Verification items for the finished model (mm, model axes). A direction names the side the tool comes from. Coordinates: 2 decimals unless noted, no trailing zeros. Loops run counter-clockwise (first coordinate to the right, second up) from the corner with the lowest first, then second, coordinate; pieces in that order, holes last. Notation, with made-up numbers: (12, 87.25) -> (46, 87.25) arc R23 ccw to (46, 95.25) -> close; hole circle Ø4 at (52.25, 61.25). An arc over 180 degrees is marked (long way). Write item = value, one per line.
```python
from build123d import *

# Parameters (mm, degrees)
F0_R         = 9.375
F1_DEPTH     = 140
F2_DEPTH     = 50
F3_SIZE      = 24
F4_T4_DEPTH  = 38.941125497
F4_T10_DEPTH = 38.941125497
F5_COUNT     = 3
F0_R_2       = 2.25
F6_DEPTH     = 10
F7_START     = 69.5
F0_R_3       = 7.5
F7_DEPTH     = 2.5
F8_DEPTH     = 25
F9_R         = 2
F10_DEPTH    = 25


# Not quite as in the source:
# - a fillet or chamfer that OpenCascade refuses, or shapes differently, is made with other operations: its cross-section is extruded or revolved along the edge and cut away or added


with BuildPart() as f1:
    # F0 (on Top) → F1 (new body)
    with BuildSketch(Plane.XY):
        with BuildLine():
            ThreePointArc((3, -9.801147892), (8.2405248619, -6.0955926701), (10.25, 0))
            ThreePointArc((10.25, 0), (7.5083287088, 6.9776428685), (0.75, 10.2225241501))
            ThreePointArc((0.75, 10.2225241501), (0, 10.25), (-0.75, 10.2225241501))
            ThreePointArc((-0.75, 10.2225241501), (-10.185896402, 1.1445586432), (-3, -9.801147892))
            ThreePointArc((-3, -9.801147892), (-1.5166961062, -10.1371659216), (-1.65e-08, -10.25))
            ThreePointArc((-1.65e-08, -10.25), (1.5166960899, -10.137165924), (3, -9.801147892))
        make_face()
        Circle(F0_R, mode=Mode.SUBTRACT)
    extrude(amount=F1_DEPTH)

    # F0 (on Top) → F2 (join)
    with BuildSketch(Plane.XY):
        with BuildLine():
            ThreePointArc((-0.75, 10.2225241501), (0, 10.25), (0.75, 10.2225241501))
            Line((0.75, 10.2225241501), (0.75, 35.2225241501))
            Line((0.75, 35.2225241501), (-0.75, 35.2225241501))
            Line((-0.75, 35.2225241501), (-0.75, 10.2225241501))
        make_face()
    extrude(amount=F2_DEPTH)

    # F3
    f3_edges = [f1.edges().sort_by_distance(p)[0] for p in [
        (0, 35.222524, 50),
    ]]
    chamfer(f3_edges, length=F3_SIZE)

    # F4: fillet of radius 1 on 2 edges, made by hand


with BuildPart() as f4_tool2:
    # F4_s3 → F4_t4 (new body)
    with BuildSketch(Plane(origin=(0, -21.1565048779, 21.1565048779), x_dir=(1, 0, 0), z_dir=(0, 0.7071067812, -0.7071067812))):
        with BuildLine():
            ThreePointArc((0.75, -42.2908619879), (0.4571067812, -42.9979687691), (-0.25, -43.2908619879))
            Line((-0.25, -43.2908619879), (-0.25, -43.3108619879))
            Line((-0.25, -43.3108619879), (0.77, -43.3108619879))
            Line((0.77, -43.3108619879), (0.77, -42.2908619879))
            Line((0.77, -42.2908619879), (0.75, -42.2908619879))
        make_face()
    extrude(amount=F4_T4_DEPTH)

    split(bisect_by=Plane.XZ.offset(-35.2225241501), keep=Keep.TOP)

    split(bisect_by=Plane.XY.offset(50), keep=Keep.BOTTOM)


with BuildPart() as f1_1:
    add(f1.part)

    # F4_t1: cut F4_tool2
    add(f4_tool2.part, mode=Mode.SUBTRACT)


with BuildPart() as f4_tool8:
    # F4_s9 → F4_t10 (new body)
    with BuildSketch(Plane(origin=(0, -21.1565048779, 21.1565048779), x_dir=(1, 0, 0), z_dir=(0, 0.7071067812, -0.7071067812))):
        with BuildLine():
            ThreePointArc((0.25, -43.2908619879), (-0.4571067812, -42.9979687691), (-0.75, -42.2908619879))
            Line((-0.75, -42.2908619879), (-0.77, -42.2908619879))
            Line((-0.77, -42.2908619879), (-0.77, -43.3108619879))
            Line((-0.77, -43.3108619879), (0.25, -43.3108619879))
            Line((0.25, -43.3108619879), (0.25, -43.2908619879))
        make_face()
    extrude(amount=F4_T10_DEPTH)

    split(bisect_by=Plane.XZ.offset(-35.2225241501), keep=Keep.TOP)

    split(bisect_by=Plane.XY.offset(50), keep=Keep.BOTTOM)


with BuildPart() as f1_2:
    add(f1_1.part)

    # F4_t7: cut F4_tool8
    add(f4_tool8.part, mode=Mode.SUBTRACT)


with BuildPart() as f5_1:
    # F5: instance of F1
    add(f1_2.part.rotate(Axis((0, 0, 0), (0, 0, -1)), 1 * 360 / F5_COUNT))


with BuildPart() as f5_2:
    # F5: instance of F1
    add(f1_2.part.rotate(Axis((0, 0, 0), (0, 0, -1)), 2 * 360 / F5_COUNT))


with BuildPart() as f1_3:
    add(f1_2.part)

    add(f5_1.part)  # F6 merges F5_1

    add(f5_2.part)  # F6 merges F5_2
    # F0 (on Top) → F6 (join)
    with BuildSketch(Plane.XY):
        with BuildLine():
            ThreePointArc((3, -13.25), (2.1213203377, -11.1286796506), (-1.65e-08, -10.25))
            ThreePointArc((-1.65e-08, -10.25), (-2.1213203494, -11.1286796623), (-3, -13.25))
            ThreePointArc((-3, -13.25), (0, -16.25), (3, -13.25))
        make_face()
        with Locations((0, -13.25)):
            Circle(F0_R_2, mode=Mode.SUBTRACT)
        with BuildLine():
            ThreePointArc((-3, -13.25), (-2.1213203494, -11.1286796623), (-1.65e-08, -10.25))
            ThreePointArc((-1.65e-08, -10.25), (-1.5166961062, -10.1371659216), (-3, -9.801147892))
            Line((-3, -9.801147892), (-3, -13.25))
        make_face()
        with BuildLine():
            Line((3, -13.25), (3, -9.801147892))
            ThreePointArc((3, -9.801147892), (1.5166960899, -10.137165924), (-1.65e-08, -10.25))
            ThreePointArc((-1.65e-08, -10.25), (2.1213203377, -11.1286796506), (3, -13.25))
        make_face()
    extrude(amount=F6_DEPTH)

    # F0 (on Top) → F7 (join)
    with BuildSketch(Plane.XY.offset(F7_START)):
        Circle(F0_R)
        Circle(F0_R_3, mode=Mode.SUBTRACT)
    extrude(amount=F7_DEPTH)

    # F0 (on Top) → F8 (join)
    with BuildSketch(Plane.XY):
        with BuildLine():
            ThreePointArc((3, -13.25), (2.1213203377, -11.1286796506), (-1.65e-08, -10.25))
            ThreePointArc((-1.65e-08, -10.25), (-2.1213203494, -11.1286796623), (-3, -13.25))
            ThreePointArc((-3, -13.25), (0, -16.25), (3, -13.25))
        make_face()
        with Locations((0, -13.25)):
            Circle(F0_R_2, mode=Mode.SUBTRACT)
        with BuildLine():
            Line((3, -13.25), (3, -9.801147892))
            ThreePointArc((3, -9.801147892), (1.5166960899, -10.137165924), (-1.65e-08, -10.25))
            ThreePointArc((-1.65e-08, -10.25), (2.1213203377, -11.1286796506), (3, -13.25))
        make_face()
        with BuildLine():
            ThreePointArc((-3, -13.25), (-2.1213203494, -11.1286796623), (-1.65e-08, -10.25))
            ThreePointArc((-1.65e-08, -10.25), (-1.5166961062, -10.1371659216), (-3, -9.801147892))
            Line((-3, -9.801147892), (-3, -13.25))
        make_face()
    extrude(amount=F8_DEPTH)

    # F9 (on Right) → F10 (cut)
    with BuildSketch(Plane.YZ):
        with Locations((0, 112.2226320051)):
            Circle(F9_R)
        with Locations((0, 101.8494740129)):
            Circle(F9_R)
    extrude(amount=-F10_DEPTH, mode=Mode.SUBTRACT)


solid = f1_3.part
```
1) Material ranges on line 1 (Y direction, x = 0, z = 123) (3 decimals); line 2 (Y direction, x = 6.5, z = 117); line 3 (Z direction, x = 8.5, y = -0.5), recorded low to high.
Ans:
line_1 = -10.25 to -9.375, 9.375 to 10.25
line_2 = -7.93 to -6.76, 6.76 to 7.93
line_3 = 69.5 to 72
2) Sectioned sample at D-D, the plane z = 119. Record the cut outline in (x, y) (3 decimals), plus the area to 3 significant figures.
Ans:
outline = circle Ø20.5 at (0, 0); hole circle Ø18.75 at (0, 0)
area = 53.9 mm2
3) Depth check by flat-ended pin: pin 1 Ø5 at (y, z) = (0, 112.22) entering from +X; pin 2 Ø9.5 at (x, y) = (0.5, 4) entering from -Z; pin 3 Ø12 at (x, z) = (11, 93.5) entering from +Y. Enter the tip coordinate at first touch or a pass-through.
Ans:
pin_1 = 10.25
pin_2 = 69.5
pin_3 = 8.95
4) Release check for a two-part mould opening along Y. For faces 4 (the face through (0.75, 23, 19)), 5 (the face through (-0.07, -16.25, 12.32)), 6 (the face through (-9.7, 1.85, 111.46)) record: pulls with the +Y half, pulls with the -Y half, needs draft (parallel to the pull), parting line crosses it, or undercut.
Ans:
face_4 = needs draft
face_5 = pulls with the -Y half
face_6 = undercut
5) Tool access check on faces 1 (the face through (3, -12, 12)), 2 (the face through (0, 8, 69.5)), 3 (the face through (0, 8, 72)). Record the directions out of +Z, -Z, +X, -X, +Y, -Y that give a thin tool (end or side, any length) a straight path to the whole face; none if there is none.
Ans:
face_1 = +Z, -Z, -Y
face_2 = -Z
face_3 = +Z
6) Sectioned sample at C-C, the plane x = 4.5. Record the cut outline in (y, z), plus the area to 3 significant figures.
Ans:
outline = (-9.21, 0) -> (-8.22, 0) -> (-8.22, 69.5) -> (-6, 69.5) -> (-6, 72) -> (-8.22, 72) -> (-8.22, 140) -> (-9.21, 140) -> close; (6, 69.5) -> (8.22, 69.5) -> (8.22, 0) -> (9.21, 0) -> (9.21, 140) -> (8.22, 140) -> (8.22, 72) -> (6, 72) -> close
area = 287 mm2
7) Sectioned sample at B-B, the plane z = 9. Record the cut outline in (x, y) (3 decimals), plus the area to 3 significant figures.
Ans:
outline = (-30.879, -16.962) -> (-30.129, -18.261) -> (-8.478, -5.761) arc R10.25 ccw to (-3, -9.801) -> (-3, -13.25) arc R3 ccw to (3, -13.25) -> (3, -9.801) arc R10.25 ccw to (8.478, -5.761) -> (30.129, -18.261) -> (30.879, -16.962) -> (9.228, -4.462) arc R10.25 ccw to (0.75, 10.223) -> (0.75, 35.223) -> (-0.75, 35.223) -> (-0.75, 10.223) arc R10.25 ccw to (-9.228, -4.462) -> close; hole circle Ø18.75 at (0, 0); hole circle Ø4.5 at (0, -13.25)
area = 183 mm2
8) Sectioned sample at A-A, the plane y = 0. Record the cut outline in (x, z) (3 decimals).
Ans:
outline = (-10.25, 0) -> (-9.375, 0) -> (-9.375, 69.5) -> (-7.5, 69.5) -> (-7.5, 72) -> (-9.375, 72) -> (-9.375, 99.849) -> (-10.25, 99.849) -> close; (-10.25, 103.849) -> (-9.375, 103.849) -> (-9.375, 110.223) -> (-10.25, 110.223) -> close; (-10.25, 114.223) -> (-9.375, 114.223) -> (-9.375, 140) -> (-10.25, 140) -> close; (7.5, 69.5) -> (9.375, 69.5) -> (9.375, 0) -> (10.25, 0) -> (10.25, 140) -> (9.375, 140) -> (9.375, 72) -> (7.5, 72) -> close
